Model file for the job. Use its own axes, mm. A direction names the side the tool comes from. Give positions to 0.01 mm unless a question says otherwise; leave off trailing zeros. Order: outer loops, then holes, each group sorted by start corner. A loop starts at its lowest first (then second) coordinate and runs counter-clockwise, first axis right, second up. Notation, with made-up numbers: (88.25, 12) - (128.25, 12) arc R23 cw to (128.25, 39) - close; hole circle Ø9 at (37.5, 37.25). An arc over 180 degrees is marked (long way). Use CSV: the item, a comma, the result in double quotes. Start each with the question number.
(1) Band-saw the part on B-B, the plane y = 11. Give the cut face in (x, z), then the cut area to 3 significant figures.
(2) Band-saw the part on C-C, the plane x = -21.5. Give the cut face in (y, z), then the cut area to 3 significant figures.
(3) Pull direction Z, two halves, no side cores. Call faces 1 (the flat face through (1, 0, -37.5)), 2 (the flat face through (0, 15, -36)), 3 (the flat face through (0, 1, 35)): +Z half, -Z half, draft (parallel to the pull), parting line (faces both ways), or undercut.
(4) Probe L1, parallel to Z at x = 57.5, y = 3.75; L2, parallel to X at y = -7, z = 30; L3, parallel to Y at x = -16, z = 14.5. List the from-to ranges inside material, lowest first.
(5) Drop flat-ended pins along their axis: pin 1 Ø14 at (y, z) = (5, -10) entering from -X; pin 2 Ø1 at (x, z) = (-21.5, 25) entering from +Y. Give the stop position or say it passes through.
(6) Band-saw the part on A-A, the plane z = 4. Give the cut face in (x, y), then the cut area to 3 significant figures.
(7) Tool access for faces 4 (the flat face through (-2, -12.5, 0)), 5 (the flat face through (75, 0, 1)): list every direction of +Z, -Z, +X, -X, +Y, -Y with a clear straight run to the whole face (end or side of a thin tool).
from build123d import *

# Parameters (mm, degrees)
BOSS_EXTRUDE1_DEPTH = 15
BOSS_EXTRUDE2_START = -15
SKETCH2_3_W         = 145
SKETCH2_3_H         = 70
SKETCH2_3_W_2       = 2.5
BOSS_EXTRUDE2_DEPTH = 2.5


with BuildPart() as part:
    # Sketch2 → Boss-Extrude1 (new, symmetric)
    with BuildSketch(Plane(origin=(0, 0, 0), x_dir=(1, 0, 0), z_dir=(0, 1, 0))):
        Polygon((-75, 35), (-72.5, 35), (72.5, 35), (72.5, -35), (-72.5, -35), (-75, -35), (-75, -37.5), (75, -37.5), (75, 37.5), (-75, 37.5), align=None)
    extrude(amount=BOSS_EXTRUDE1_DEPTH, both=True)

    # Sketch2<3> → Boss-Extrude2 (add)
    with BuildSketch(Plane(origin=(0, 0, 0), x_dir=(1, 0, 0), z_dir=(0, 1, 0)).offset(BOSS_EXTRUDE2_START)):
        Rectangle(SKETCH2_3_W, SKETCH2_3_H)
        with Locations((-73.75, 0)):
            Rectangle(SKETCH2_3_W_2, SKETCH2_3_H)
    extrude(amount=BOSS_EXTRUDE2_DEPTH)


solid = part.part
Answer block:
1,outline,"(-75, -37.5) - (75, -37.5) - (75, 37.5) - (-75, 37.5) - (-75, 35) - (72.5, 35) - (72.5, -35) - (-75, -35) - close"
1,area,"925 mm2"
2,outline,"(-15, -37.5) - (15, -37.5) - (15, -35) - (-12.5, -35) - (-12.5, 35) - (15, 35) - (15, 37.5) - (-15, 37.5) - close"
2,area,"325 mm2"
3,face 1,"-Z half"
3,face 2,"draft"
3,face 3,"undercut"
4,L1,"z = -37.5 to -35, 35 to 37.5"
4,L2,"x = 72.5 to 75"
4,L3,"y = -15 to -12.5"
5,pin 1,"stops at x = 72.5"
5,pin 2,"stops at y = -12.5"
6,outline,"(-75, -15) - (75, -15) - (75, 15) - (72.5, 15) - (72.5, -12.5) - (-75, -12.5) - close"
6,area,"444 mm2"
7,face 4,"-X, +Y"
7,face 5,"+Z, -Z, +X, +Y, -Y"
